```python
from build123d import *

# Parameters (mm, degrees)
SKETCH001_W  = 15
SKETCH001_H  = 20
PAD001_DEPTH = 14
SKETCH002_R  = 4.5
PAD002_DEPTH = 10
SKETCH003_R  = 3.15
PAD003_DEPTH = 12
FILLET_R     = 2


with BuildPart() as part:
    # Sketch001 → Pad001 (new body)
    with BuildSketch(Plane.XZ):
        Rectangle(SKETCH001_W, SKETCH001_H)
    extrude(amount=PAD001_DEPTH)

    # Sketch002 → Pad002 (join)
    with BuildSketch(Plane(origin=(0, -14, 1), x_dir=(1, 0, 0), z_dir=(0, -1, 0))):
        Circle(SKETCH002_R)
    extrude(amount=PAD002_DEPTH)

    # Sketch003 → Pad003 (join)
    with BuildSketch(Plane(origin=(0, -24, 1), x_dir=(1, 0, 0), z_dir=(0, -1, 0))):
        Circle(SKETCH003_R)
    extrude(amount=PAD003_DEPTH)

    # Fillet
    fillet_edges = [part.edges().sort_by_distance(p)[0] for p in [
        (-7.5, -7, 10),
        (0, -14, 10),
        (-7.5, -14, 0),
        (7.5, -14, 0),
        (-7.5, -7, -10),
        (0, -14, -10),
        (7.5, -7, -10),
        (7.5, -7, 10),
    ]]
    fillet(fillet_edges, radius=FILLET_R)


with BuildPart() as part_1:
    # Body001 placement: moved
    add(part.part.moved(Location((0, -413, 17))))


solid = part_1.part
```
The model under review builds one solid part; all positions refer to its coordinate system, in mm. A direction names the side the tool comes from. Round coordinates to 2 decimals unless told otherwise and drop trailing zeros. Loops run counter-clockwise (first coordinate to the right, second up) from the corner with the lowest first, then second, coordinate; pieces in that order, holes last. Notation, with made-up numbers: (74, 44) -> (115, 44) arc R24 ccw to (115, 79) -> close; hole circle Ø10 at (60, -11.5). An arc over 180 degrees is marked (long way). Answer as a JSON object with one key per item and string values. Group by question number.
1) We need section B-B on x = 2.5. Write out the cut boundary in (y, z).
2) For pin 1 Ø5 at (x, z) = (-3.5, 19.5) entering from -Y; pin 2 Ø1.5 at (x, y) = (3, -442.5) entering from +Z; pin 3 Ø8 at (y, z) = (-434, 20) entering from -X, all flat-tipped, find the tip position at first contact; note any pin that passes through.
3) We need section C-C on y = -433. Write out the cut boundary in (x, z), then the cut area to 3 significant figures.
4) For faces 1 (the face through (-4, -427, 15)), 2 (the face through (6.9, -419.08, 7.57)), list the 3-axis set-ups (+Z, -Z, +X, -X, +Y, -Y) from which the entire face can be reached by the end or side of a thin tool; tool diameter is ignored.
5) We need section D-D on z = 10.25. Write out the cut boundary in (x, y).
6) For line 1 (Y direction, x = 3.25, z = 21.5); line 2 (Y direction, x = -6.25, z = 24); line 3 (Z direction, x = -1.5, y = -445), list the stretches that pass through material, from the lowest coordinate up. Write a range as [from, to].
7) We need section A-A on z = 18. Write out the cut boundary in (x, y).
Result set:
{
 "1": {"outline": "(-449, 16.08) -> (-437, 16.08) -> (-437, 14.26) -> (-427, 14.26) -> (-427, 9) arc R2 ccw to (-425, 7) -> (-413, 7) -> (-413, 27) -> (-425, 27) arc R2 ccw to (-427, 25) -> (-427, 21.74) -> (-437, 21.74) -> (-437, 19.92) -> (-449, 19.92) -> close"},
 "2": {"pin 1": "y = -449", "pin 2": "z = 20.2", "pin 3": "x = -4.5"},
 "3": {"outline": "circle Ø9 at (0, 18)", "area": "63.6 mm²"},
 "4": {"face 1": "-Y", "face 2": "-Z, +X, +Y, -Y"},
 "5": {"outline": "(-7.5, -425) arc R2 ccw to (-5.5, -427) -> (5.5, -427) arc R2 ccw to (7.5, -425) -> (7.5, -413) -> (-7.5, -413) -> close"},
 "6": {"line 1": "[-427, -413]", "line 2": "[-426.85, -413]", "line 3": "[15.23, 20.77]"},
 "7": {"outline": "(-7.5, -425) arc R2 ccw to (-5.5, -427) -> (-4.5, -427) -> (-4.5, -437) -> (-3.15, -437) -> (-3.15, -449) -> (3.15, -449) -> (3.15, -437) -> (4.5, -437) -> (4.5, -427) -> (5.5, -427) arc R2 ccw to (7.5, -425) -> (7.5, -413) -> (-7.5, -413) -> close"}
}
